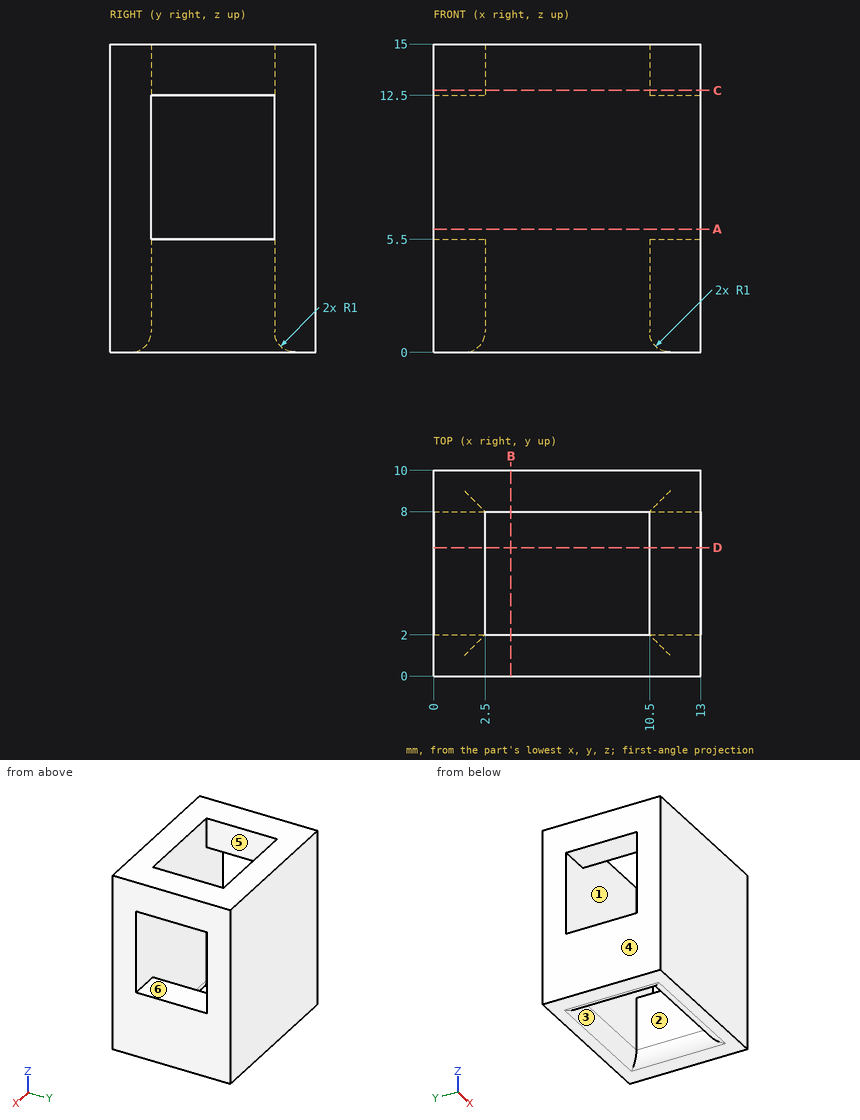
Part print with two shaded views. Sizes in mm from the minimum x, y, z corner. A direction names the side the tool comes from. Round coordinates to 2 decimals unless told otherwise and drop trailing zeros. Loops run counter-clockwise (first coordinate to the right, second up) from the corner with the lowest first, then second, coordinate; pieces in that order, holes last. Notation, with made-up numbers: (15, 70) - (67, 70) arc R20 cw to (67, 105) - close; hole circle Ø10 at (-28.5, 50.25). An arc over 180 degrees is marked (long way). Answer as a JSON object with one key per item and string values.
Item 1: Tool access for the marked faces 1, 2 and 3: list every direction of +Z, -Z, +X, -X, +Y, -Y with a clear straight run to the whole face (end or side of a thin tool).
Output:
{"face 1": "none", "face 2": "+Z, -Z", "face 3": "-Z"}
Item 2: Pin check, flat tip, straight feed: pin 1 (3 mm diameter, centred on y = 5.5, z = 14, fed in from -X). Stop position of the tip, or through.
Output:
{"pin 1": "x = 0"}
Item 3: Band-saw the part on D-D on y = 6.25. List the corners of the cut face in (x, z).
Output:
{"outline": "(0, 0) - (1.5, 0) arc R1 ccw to (2.5, 1) - (2.5, 5.5) - (0, 5.5) - close; (0, 12.5) - (2.5, 12.5) - (2.5, 15) - (0, 15) - close; (10.5, 1) arc R1 ccw to (11.5, 0) - (13, 0) - (13, 5.5) - (10.5, 5.5) - close; (10.5, 12.5) - (13, 12.5) - (13, 15) - (10.5, 15) - close"}
Item 4: Band-saw the part on B-B on x = 3.75. List the corners of the cut face in (y, z), plus the area to 3 significant figures.
Output:
{"outline": "(0, 0) - (1, 0) arc R1 ccw to (2, 1) - (2, 15) - (0, 15) - close; (8, 1) arc R1 ccw to (9, 0) - (10, 0) - (10, 15) - (8, 15) - close", "area": "59.6 mm2"}
Item 5: Wall check: L1, parallel to Y at x = 8.75, z = 1.5; L2, parallel to X at y = 6, z = 13.5; L3, parallel to Z at x = 0.5, y = 7.75. Give the ranges that are in metal, low to high.
Output:
{"L1": "0 to 2, 8 to 10", "L2": "0 to 2.5, 10.5 to 13", "L3": "0 to 5.5, 12.5 to 15"}
Item 6: Band-saw the part on C-C on z = 12.75. List the corners of the cut face in (x, y), plus the area to 3 significant figures.
Output:
{"outline": "(0, 0) - (13, 0) - (13, 10) - (0, 10) - close; hole (2.5, 2) - (10.5, 2) - (10.5, 8) - (2.5, 8) - close", "area": "82.0 mm2"}
Item 7: Band-saw the part on A-A on z = 6. List the corners of the cut face in (x, y).
Output:
{"outline": "(0, 0) - (13, 0) - (13, 2) - (0, 2) - close; (0, 8) - (13, 8) - (13, 10) - (0, 10) - close"}
Item 8: Pull direction X, two halves, no side cores. Call the marked faces 4, 5 and 6: pulls with the +X half, pulls with the -X half, needs draft (parallel to the pull), parting line crosses it, or undercut.
Output:
{"face 4": "pulls with the -X half", "face 5": "undercut", "face 6": "needs draft"}
